Geometry check sheet. Reference: the model listing, model coordinates, mm. A direction names the side the tool comes from. Coordinates: 2 decimals unless noted, no trailing zeros. Loops run counter-clockwise (first coordinate to the right, second up) from the corner with the lowest first, then second, coordinate; pieces in that order, holes last. Notation, with made-up numbers: (-8.75, -18) - (5.25, -18) arc R19 cw to (5.25, 9) - close; hole circle Ø7 at (-36, -36). An arc over 180 degrees is marked (long way). Write each question's results on one line, items separated by ' | '. Start each with the question number.
(1) Sectioned sample at D-D (z = -9). Enter the section's corners in (x, y).
(2) Go/stop test with flat-tipped pins: pin 1 Ø5 at (x, y) = (17, -27.5) entering from -Z; pin 2 Ø3 at (x, z) = (9, -28) entering from +Y; pin 3 Ø8 at (x, y) = (7, 12) entering from +Z. Record where each tip stops, or that it passes through.
(3) Sectioned sample at B-B (x = -2.5). Enter the section's corners in (y, z).
(4) Mould release check, pull along X, two halves, no side actions. Record for faces 1 (the face through (-8.997, 7.003, 8.541)), 2 (the face through (-14.53, -39.13, -43)), 3 (the face through (0.77, 25.61, 3.13)), 4 (the face through (26.416, -17, 1)): pulls with the +X half, pulls with the -X half, needs draft (parallel to the pull), parting line crosses it, or undercut.
(5) Sectioned sample at A-A (z = -40.64). Enter the section's corners in (x, y), plus the area to 3 significant figures.
(6) Access from +Z, -Z, +X, -X, +Y, -Y to the whole of each face (thin tool, end or side, straight path). Record for faces 5 (the face through (17.536, -39.13, -42.648)), 6 (the face through (1, -34.121, -25)).
(7) Sectioned sample at C-C (y = -31.5). Enter the section's corners in (x, z).
(8) Material ranges on probe 1 along X at (y, z) = (-41.25, -40.64); probe 2 along Y at (x, z) = (-19, -37.5); probe 3 along Z at (x, y) = (10.5, 24), recorded low to high.
Autodesk Inventor part; units mm, degrees
ref_plane "YZ Plane" through (0, 0, 0) normal (1, 0, 0) x (0, 1, 0)
ref_plane "XZ Plane" through (0, 0, 0) normal (0, 1, 0) x (-1, 0, 0)
ref_plane "XY Plane" through (0, 0, 0) normal (0, 0, 1) x (1, 0, 0)
sketch "Sketch1" plane through (0, 0, 0) normal (0, 0, 1) x (1, 0, 0)
  circle A0 centre (1.016, 27.4993) radius 1.905
  arc A1 (-3.2174, 19.2546) -> (-0.4706, 18.1168) centre (1.016, 25.5904) ccw
  circle A2 centre (1.016, 25.5904) radius 7.62
  arc A3 (-0.4706, -2.0514) -> (-3.2174, -3.1892) centre (1.016, -9.525) ccw
  arc A4 (2.5026, -16.9986) -> (5.2494, -15.8608) centre (1.016, -9.525) ccw
  circle A5 centre (1.016, -9.525) radius 7.62
  line L0 (1.016, -1.905) -> (1.016, 17.9704)
  circle A6 centre (1.016, 8.0327) radius 9.525
  line L1 (0, 16.0654) -> (2.032, 16.0654)
  line L2 (2.032, 0) -> (0, 0)
  circle A7 centre (-7.874, 8.0327) radius 9.525
  line L3 (26.416, 41.9773) -> (-24.384, 41.9773)
  line L4 (-24.384, -44.2811) -> (-24.384, 41.9773)
  line L5 (26.416, -44.2811) -> (26.416, 41.9773)
  line L6 (-75.184, -44.2811) -> (77.216, -44.2811)
  line L7 (1.016, 8.0327) -> (-47.2731, 8.0327)
  circle A8 centre (-24.384, 8.0327) radius 21.5247
  circle A9 centre (1.016, -9.525) radius 1.905
  circle A10 centre (-7.874, 8.0327) radius 1.905
  point P0 (0, 0)
  dimension "d0" = 19.05
  dimension "d1" = 19.05
  dimension "d2" = 8.89
  dimension "d3" = 3.81
  dimension "d4" = 3.81
  dimension "d5" = 3.81
  dimension "d32" = 71.7804
  dimension "d33" = 44.2811
  dimension "d34" = 25.4
  dimension "d35" = 0
  dimension "d36" = 0
  dimension "d37" = 86.2584
extrude "Extrusion1" add sketch "Sketch1" along normal blind 6.35 contours A2 A1 | A5 A4 A3 | A6 A7 A8 L4 L3 L5 L6 | A7 A8 A6 | A6 A8 L7 L0 A7 | L0 A7 | A8 A7 L7 A10 A6 | A6 A10 L7 A8 | A8 L4 L7 A7 | L7 A8 A6 A7 L0 | L7 A10 A6 A8 | L7 L4 A8 A7 | A7 A8 A6 A10 L7 | A6 A8 A7 | A9
sketch "Sketch2" plane through (0, 0, 6.35) normal (0, 0, 1) x (1, 0, 0)
  line L0 (-3.429, -3.0002) -> (13.2364, -3.0002)
  line L1 (13.2364, -3.0002) -> (13.2364, 18.7074)
  line L2 (13.2364, 18.7074) -> (-3.429, 18.7074)
  line L3 (-3.429, 18.7074) -> (-3.429, -3.0002)
  point P0 (0, 0)
extrude "Extrusion2" add sketch "Sketch2" against normal blind 6.35
sketch "Sketch3" plane through (0, 0, 0) normal (0, 0, -1) x (-1, 0, 0)
  line L0 (24.384, 41.9773) -> (24.384, -44.2811)
  line L1 (-26.416, -44.2811) -> (24.384, -44.2811)
  line L2 (24.384, -44.2811) -> (24.384, -34.1211)
  line L3 (24.384, -34.1211) -> (-26.416, -34.1211)
  line L4 (-26.416, -34.1211) -> (-26.416, -44.2811)
  point P0 (0, 0)
  dimension "d10" = 10.16
extrude "Extrusion3" add sketch "Sketch3" along normal blind 50.8
sketch "Sketch4" plane through (-24.384, -34.1211, 0) normal (0, 1, 0) x (1, 0, 0)
  circle A0 centre (40.64, 40.64) radius 2.3813
  circle A1 centre (10.16, 40.64) radius 2.3813
  line L0 (50.8, 0) -> (0, 0)
  line L1 (0, 50.8) -> (50.8, 50.8)
  line L2 (50.8, 0) -> (50.8, 50.8)
  line L3 (0, 0) -> (0, 50.8)
  point P0 (24.384, 0)
  dimension "d13" = 4.7625
  dimension "d14" = 4.7625
  dimension "d17" = 10.16
  dimension "d18" = 10.16
  dimension "d19" = 10.16
  dimension "d20" = 10.16
extrude "Extrusion4" cut sketch "Sketch4" against normal up to next contours A0 | A1
sketch "Sketch5" plane through (0, 0, 6.35) normal (0, 0, 1) x (1, 0, 0)
  circle A0 centre (-7.874, 8.0327) radius 1.905
  point P0 (0, 0)
extrude "Extrusion5" add sketch "Sketch5" against normal blind 6.35
sketch "Sketch6" plane through (0, 0, 6.35) normal (0, 0, 1) x (1, 0, 0)
  circle A0 centre (-7.874, 8.0327) radius 1.524
  point P0 (0, 0)
  dimension "d27" = 3.048
  dimension "d28" = 8.0327
  dimension "d29" = 7.874
extrude "Extrusion6" add sketch "Sketch6" along normal blind 4.445
properties part number "Middle Gear Frame"
Outcome:
1) outline: (-24.38, -44.28) - (26.42, -44.28) - (26.42, -34.12) - (-24.38, -34.12) - close
2) pin 1: stops at z = 0 | pin 2: stops at y = -34.12 | pin 3: stops at z = 6.35
3) outline: (-44.28, -50.8) - (-34.12, -50.8) - (-34.12, 0) - (41.98, 0) - (41.98, 6.35) - (-44.28, 6.35) - close
4) face 1: parting line crosses it | face 2: undercut | face 3: undercut | face 4: pulls with the +X half
5) outline: (-24.38, -44.28) - (-16.61, -44.28) - (-16.61, -34.12) - (-24.38, -34.12) - close; (-11.84, -44.28) - (13.87, -44.28) - (13.87, -34.12) - (-11.84, -34.12) - close; (18.64, -44.28) - (26.42, -44.28) - (26.42, -34.12) - (18.64, -34.12) - close | area: 419 mm2
6) face 5: +Y, -Y | face 6: -Z, +X, -X, +Y
7) outline: (-24.38, 0) - (26.42, 0) - (26.42, 6.35) - (-24.38, 6.35) - close
8) probe 1: x = -24.38 to -16.61, -11.84 to 13.87, 18.64 to 26.42 | probe 2: y = -44.28 to -34.12 | probe 3: z = 0 to 6.35
